Study the drawing (mm; zero at the part's minimum x, y, z) and answer. A direction names the side the tool comes from. Coordinates: 2 decimals unless noted, no trailing zeros. Write each loop counter-clockwise with the first axis right and the second up, starting at its lowest first coordinate (ties: lowest second). Pieces come first, ordered by that corner, then holes. Notation, with made-up numbers: (-8.75, 11.25) -> (-1.75, 11.25) arc R16 cw to (-1.75, 26.25) -> close; hole circle Ø7 at (-15.5, -35). An arc over 180 degrees is marked (long way). Answer in a Markdown table with one row per item. Add a question column.
Item 1: Section D-D on y = 2.5 is taken. Write down the section's boundary in (x, z).
Item 2: Section C-C on y = 5.5 is taken. Write down the section's boundary in (x, z), then the cut area to 3 significant figures.
Item 3: Section A-A on z = 13.75 is taken. Count the separate pieces of the cut face and the enclosed holes in it, then the cut area to 3 significant figures.
Item 4: Which of the six approach directions +Z, -Z, +X, -X, +Y, -Y give full straight-line access (tool end or side, diameter ignored) to the marked faces 1 and 2?
Item 5: Section B-B on x = 5 is taken. Write down the section's boundary in (y, z), then the cut area to 3 significant figures.
Item 6: Straight lines are drawn through the part: line 1 (Y direction, x = 47.8, z = 14.4); line 2 (Z direction, x = 2, y = 8.75); line 3 (X direction, y = 3, z = 6.25). For each, find the intervals that lie inside material, in ascending order. Write a range as from..to.
Item 7: For a pull along X with two mould halves and no side action, classify the marked faces 3, 4 and 5 as +X half, -X half, draft (parallel to the pull), parting line (faces both ways), or undercut.
Item 8: Given pin 1 Ø4.5 at (x, y) = (47, 3) entering from -Z; pin 2 Ø2 at (x, y) = (36, 3.5) entering from -Z; pin 3 Ø2.5 at (x, y) = (47.8, 4.5) entering from +Z; pin 4 Ø5 at (x, y) = (35, 2) entering from -Z, each flat-ended and moving along its own axis, determine where each tip first touches the part or whether it passes through.
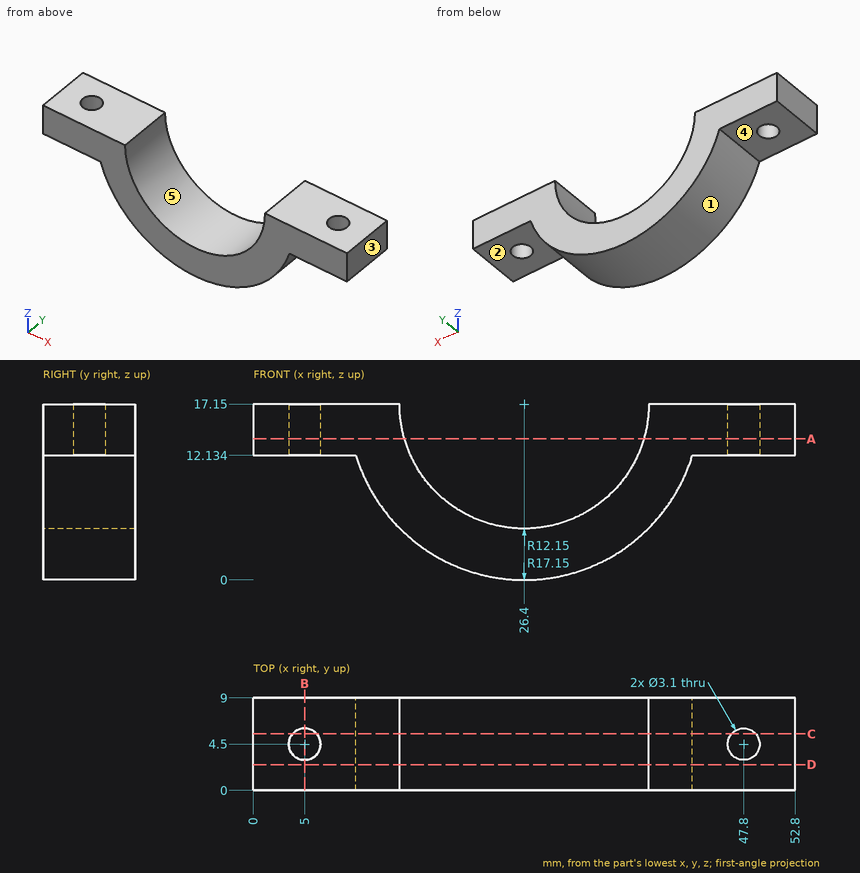
Results below:
| question | item | result |
|---|---|---|
| 1 | outline | (0, 12.13) -> (10, 12.13) arc R17.15 ccw to (42.8, 12.13) -> (52.8, 12.13) -> (52.8, 17.15) -> (38.55, 17.15) arc R12.15 cw to (14.25, 17.15) -> (0, 17.15) -> close |
| 2 | outline | (0, 12.13) -> (3.82, 12.13) -> (3.82, 17.15) -> (0, 17.15) -> close; (6.18, 12.13) -> (10, 12.13) arc R17.15 ccw to (42.8, 12.13) -> (46.62, 12.13) -> (46.62, 17.15) -> (38.55, 17.15) arc R12.15 cw to (14.25, 17.15) -> (6.18, 17.15) -> close; (48.98, 12.13) -> (52.8, 12.13) -> (52.8, 17.15) -> (48.98, 17.15) -> close |
| 2 | area | 302 mm2 |
| 3 | separate pieces | 2 |
| 3 | enclosed holes | 2 |
| 3 | area | 250 mm2 |
| 4 | face 1 | -Z, +Y, -Y |
| 4 | face 2 | -Z, +X, +Y, -Y |
| 5 | outline | (0, 12.13) -> (2.95, 12.13) -> (2.95, 17.15) -> (0, 17.15) -> close; (6.05, 12.13) -> (9, 12.13) -> (9, 17.15) -> (6.05, 17.15) -> close |
| 5 | area | 29.6 mm2 |
| 6 | line 1 | y = 0..2.95, 6.05..9 |
| 6 | line 2 | z = 12.13..17.15 |
| 6 | line 3 | x = 13.16..21.03, 31.77..39.64 |
| 7 | face 3 | +X half |
| 7 | face 4 | draft |
| 7 | face 5 | undercut |
| 8 | pin 1 | stops at z = 12.13 |
| 8 | pin 2 | stops at z = 2.31 |
| 8 | pin 3 | passes through |
| 8 | pin 4 | stops at z = 1.12 |
